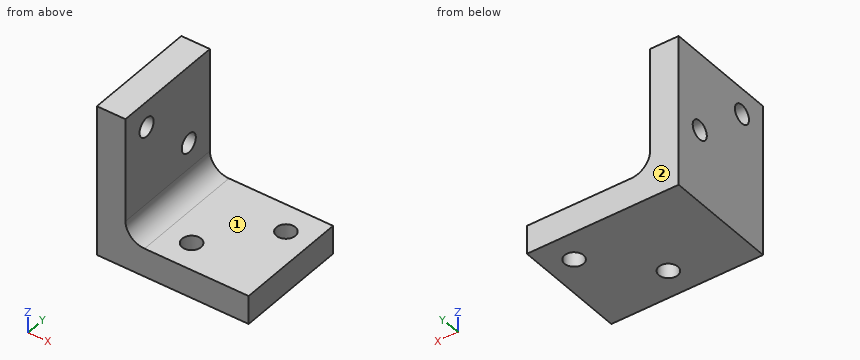
```python
from build123d import *

# Parameters (mm, degrees)
F0_W     = 50.6476
F0_H     = 50.6476
F1_DEPTH = 38.1
F3_DEPTH = 38.101
F4_R     = 3.175
F5_DEPTH = 9.526
F6_R     = 3.175
F7_DEPTH = 9.526


with BuildPart() as f1:
    # F0 (on Front) → F1 (new body)
    with BuildSketch(Plane.XZ):
        with Locations((25.3238, 25.3238)):
            Rectangle(F0_W, F0_H)
    extrude(amount=F1_DEPTH)

    # F2 (on face) → F3 (cut, through all)
    with BuildSketch(Plane.XZ.offset(38.1)):
        with BuildLine():
            Line((50.6476, 9.525), (50.6476, 50.6476))
            Line((50.6476, 50.6476), (9.525, 50.6476))
            Line((9.525, 50.6476), (9.525, 15.875))
            ThreePointArc((9.525, 15.875), (11.384872, 11.384872), (15.875, 9.525))
            Line((15.875, 9.525), (50.6476, 9.525))
        make_face()
    extrude(amount=-F3_DEPTH, mode=Mode.SUBTRACT)

    # F4 (on face) → F5 (cut, through all)
    with BuildSketch(Plane.XY.offset(9.525)):
        with Locations((24.56815, -28.575)):
            Circle(F4_R)
        with Locations((41.95445, -9.525)):
            Circle(F4_R)
    extrude(amount=-F5_DEPTH, mode=Mode.SUBTRACT)

    # F6 (on face) → F7 (cut, through all)
    with BuildSketch(Plane.YZ.offset(9.525)):
        with Locations((-28.575, 41.95445)):
            Circle(F6_R)
        with Locations((-9.525, 24.56815)):
            Circle(F6_R)
    extrude(amount=-F7_DEPTH, mode=Mode.SUBTRACT)


solid = f1.part
```
Source: CAD feature listing. Evaluate the final solid. Frame: model axes, mm. Face numbers are marked on the shaded views. A direction names the side the tool comes from. Give positions to 0.01 mm unless a question says otherwise; leave off trailing zeros. Loops run counter-clockwise (first coordinate to the right, second up) from the corner with the lowest first, then second, coordinate; pieces in that order, holes last. Notation, with made-up numbers: M -1.5,-10.75 L 40.5,-10.75 A16 ccw 40.5,11.25 Z; hole C -9.5,-7 d11. An arc over 180 degrees is marked long. Put each result on its own line as item: value.
Q1. Reachability of the marked faces 1 and 2 from +Z, -Z, +X, -X, +Y, -Y: full face, straight path, thin tool, end or side. Return the list, or none.
Response values:
face 1: +Z, +X, +Y, -Y
face 2: +Z, -Z, +X, -X, +Y
Q2. Section D-D (y = -7.5). Return the cut outline in (x, z) (3 decimals), and give its area (3 significant figures).
Response values:
outline: M 0,0 L 39.509,0 L 39.509,9.525 L 15.875,9.525 A6.35 cw 9.525,15.875 L 9.525,22.123 L 0,22.123 Z; M 0,27.014 L 9.525,27.014 L 9.525,50.648 L 0,50.648 Z; M 44.4,0 L 50.648,0 L 50.648,9.525 L 44.4,9.525 Z
area: 790 mm²
Q3. Section C-C (z = 29.5). Return the cut outline in (x, y) (3 decimals).
Response values:
outline: M 0,-38.1 L 9.525,-38.1 L 9.525,0 L 0,0 Z
Q4. Pin query (flat end, axial travel): P1, Ø3, axis at x = 20, y = -18, coming from the +Z side (3 decimals); P2, Ø10.5, axis at y = -18, z = 34.5, coming from the +X side (3 decimals). Return the tip coordinate at first contact, or that it passes through.
Response values:
P1: stops at z = 9.525
P2: stops at x = 9.525
Q5. Section A-A (y = -15.5). Return the cut outline in (x, z) (3 decimals), and give its area (3 significant figures).
Response values:
outline: M 0,0 L 50.648,0 L 50.648,9.525 L 15.875,9.525 A6.35 cw 9.525,15.875 L 9.525,50.648 L 0,50.648 Z
area: 883 mm²
Q6. Section B-B (x = 23). Return the cut outline in (y, z) (3 decimals), and give its area (3 significant figures).
Response values:
outline: M -38.1,0 L -31.336,0 L -31.336,9.525 L -38.1,9.525 Z; M -25.814,0 L 0,0 L 0,9.525 L -25.814,9.525 Z
area: 310 mm²
Q7. Line query: probe 1 along Z at (x, y) = (20, -4) (3 decimals); probe 2 along X at (y, z) = (-10.5, 7). Output: solid intervals per line, ascending. Write a range as [from, to].
Response values:
probe 1: z = [0, 9.525]
probe 2: x = [0, 38.93], [44.98, 50.65]
